Verification items for the finished model (mm, model axes). Give positions to 0.01 mm unless a question says otherwise; leave off trailing zeros. Order: outer loops, then holes, each group sorted by start corner. A loop starts at its lowest first (then second) coordinate and runs counter-clockwise, first axis right, second up. Notation, with made-up numbers: (77, -31) -> (131, -31) arc R16 cw to (131, -16) -> close; hole circle Ø11 at (-10, -26.5). An arc over 180 degrees is marked (long way). One line per question, with ' | ' between items. Start each with the question number.
Q1. Material ranges on probe 1 along X at (y, z) = (49.5, 1); probe 2 along X at (y, z) = (-35, 5.5); probe 3 along Y at (x, z) = (-40, 2.25), recorded low to high. Write a range as [from, to].
Q2. Section check B-B on z = 1.5. Record the cut outline in (x, y), plus the area to 3 significant figures.
Q3. Section check C-C on x = -51. Record the cut outline in (y, z), plus the area to 3 significant figures.
Q4. Section check A-A on y = -45. Record the cut outline in (x, z), plus the area to 3 significant figures.
Q5. Go/stop test with flat-tipped pins: pin 1 (1.5 mm diameter, centred on x = -55, z = 2, fed in from -Y); pin 2 (1.9 mm diameter, centred on x = -5, z = 4, fed in from +Y); pin 3 (12 mm diameter, centred on x = -10.5, y = -36.5, fed in from +Z); pin 4 (1.8 mm diameter, centred on x = 25.5, z = 4, fed in from -Y). Record where each tip stops, or that it passes through.
from build123d import *

# Parameters (mm, degrees)
F0_W     = 5.869098
F0_H     = 16.448125
F0_W_2   = 6.248793
F0_H_2   = 15.086499
F0_W_3   = 5.045854
F0_H_3   = 18.400892
F0_W_4   = 5.338394
F0_H_4   = 14.501419
F1_DEPTH = 6.35


with BuildPart() as f1:
    # F0 (on Top) → F1 (new body)
    with BuildSketch(Plane.XY):
        with Locations((24.084667, -42.334303)):
            Rectangle(F0_W, F0_H)
        Polygon((21.150118, -34.110241), (27.019216, -34.110241), (27.019216, 41.812751), (20.770423, 41.812751), (-59.093311, 41.812751), (-64.431705, 41.812751), (-64.431705, -34.110241), (-59.385851, -34.110241), align=None)
        with Locations((23.894819, 49.356)):
            Rectangle(F0_W_2, F0_H_2)
        with Locations((-61.908778, -43.310687)):
            Rectangle(F0_W_3, F0_H_3)
        with Locations((-61.762508, 49.06346)):
            Rectangle(F0_W_4, F0_H_4)
    extrude(amount=F1_DEPTH)


solid = f1.part
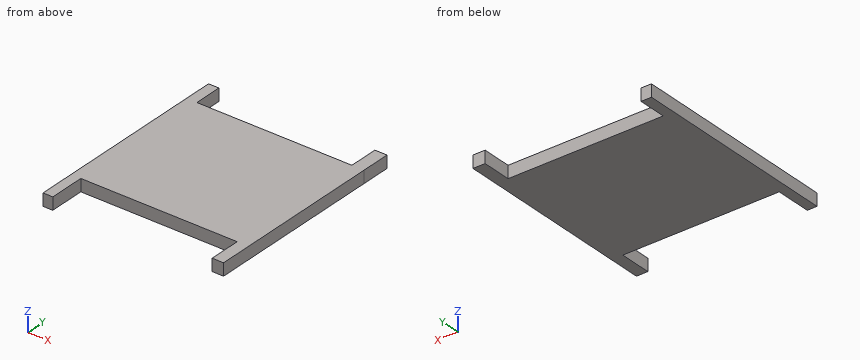
Filled in:
1) probe 1: [-64.43, -59.09], [20.77, 27.02] | probe 2: [-64.43, -59.39], [21.15, 27.02] | probe 3: [-34.11, 41.81]
2) outline: (-64.43, -52.51) -> (-59.39, -52.51) -> (-59.39, -34.11) -> (21.15, -34.11) -> (21.15, -50.56) -> (27.02, -50.56) -> (27.02, 56.9) -> (20.77, 56.9) -> (20.77, 41.81) -> (-59.09, 41.81) -> (-59.09, 56.31) -> (-64.43, 56.31) -> close | area: 7,300 mm²
3) outline: (-34.11, 0) -> (41.81, 0) -> (41.81, 6.35) -> (-34.11, 6.35) -> close | area: 482 mm²
4) outline: (-64.43, 0) -> (-59.39, 0) -> (-59.39, 6.35) -> (-64.43, 6.35) -> close; (21.15, 0) -> (27.02, 0) -> (27.02, 6.35) -> (21.15, 6.35) -> close | area: 69.3 mm²
5) pin 1: y = -34.11 | pin 2: y = 41.81 | pin 3: z = 6.35 | pin 4: y = -50.56
